Source: three-view drawing plus pictorial views. Frame: mm from the lowest corner of the part. A direction names the side the tool comes from. Round coordinates to 2 decimals unless told otherwise and drop trailing zeros. Order: outer loops, then holes, each group sorted by start corner. A loop starts at its lowest first (then second) coordinate and runs counter-clockwise, first axis right, second up. Notation, with made-up numbers: (13, -34.5) - (44, -34.5) arc R34 cw to (44, 4.5) - close; hole circle Ø9 at (56, 2). An arc over 180 degrees is marked (long way). One line per item, written item: value. Start each with the question number.
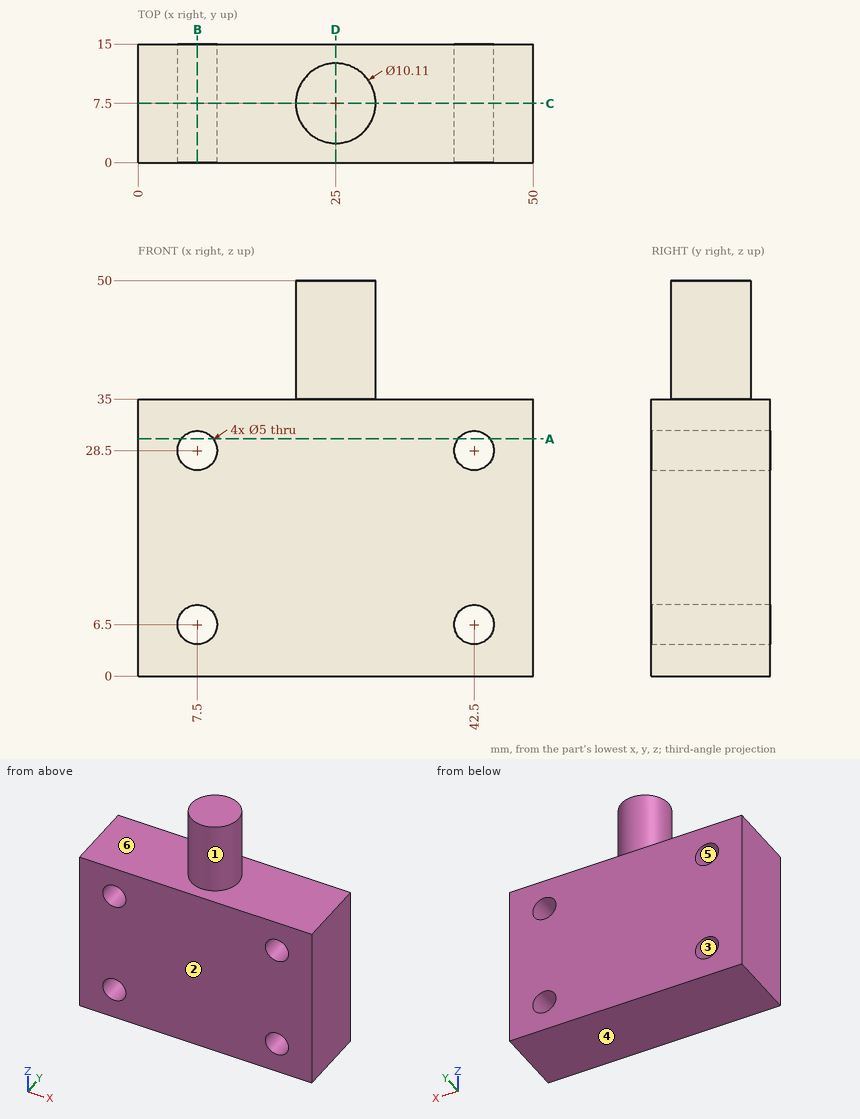
Item 1: Section query A-A on z = 30. Return loops of the section in (x, y), and give its area (3 significant figures).
Item 2: Line query: L1, parallel to X at y = 11.5, z = 6.5; L2, parallel to X at y = 7.25, z = 7; L3, parallel to Z at x = 44, y = 4.75. Output: solid intervals per line, ascending.
Item 3: Section query D-D on x = 25. Return loops of the section in (y, z) (3 decimals), and give its area (3 significant figures).
Item 4: Section query C-C on y = 7.5. Return loops of the section in (x, z) (3 decimals).
Item 5: Pull-direction query (Z, two-part tool) for the marked faces 3, 4, 5 and 6; classes: released by +Z, released by -Z, zero draft, split by the parting line, or undercut.
Item 6: Section query B-B on x = 7.5. Return loops of the section in (y, z), and give its area (3 significant figures).
Item 7: Reachability of the marked faces 1 and 2 from +Z, -Z, +X, -X, +Y, -Y: full face, straight path, thin tool, end or side. Return the list, or none.
Geometry results:
1. outline: (0, 0) - (5.5, 0) - (5.5, 15) - (0, 15) - close; (9.5, 0) - (40.5, 0) - (40.5, 15) - (9.5, 15) - close; (44.5, 0) - (50, 0) - (50, 15) - (44.5, 15) - close
1. area: 630 mm^2
2. L1: x = 0 to 5, 10 to 40, 45 to 50
2. L2: x = 0 to 5.05, 9.95 to 40.05, 44.95 to 50
2. L3: z = 0 to 4.5, 8.5 to 26.5, 30.5 to 35
3. outline: (0, 0) - (15, 0) - (15, 35) - (12.555, 35) - (12.555, 50) - (2.445, 50) - (2.445, 35) - (0, 35) - close
3. area: 677 mm^2
4. outline: (0, 0) - (50, 0) - (50, 35) - (30.055, 35) - (30.055, 50) - (19.945, 50) - (19.945, 35) - (0, 35) - close; hole circle Ø5 at (7.5, 6.5); hole circle Ø5 at (7.5, 28.5); hole circle Ø5 at (42.5, 6.5); hole circle Ø5 at (42.5, 28.5)
5. face 3: undercut
5. face 4: released by -Z
5. face 5: undercut
5. face 6: released by +Z
6. outline: (0, 0) - (15, 0) - (15, 4) - (0, 4) - close; (0, 9) - (15, 9) - (15, 26) - (0, 26) - close; (0, 31) - (15, 31) - (15, 35) - (0, 35) - close
6. area: 375 mm^2
7. face 1: +Z
7. face 2: +Z, -Z, +X, -X, -Y
